Work out the finished part from the listing and answer in its coordinate system (mm). Face numbers are marked on the shaded views. Coordinates: 2 decimals unless noted, no trailing zeros. Order: outer loops, then holes, each group sorted by start corner. A loop starts at its lowest first (then second) coordinate and runs counter-clockwise, first axis right, second up. Notation, with made-up numbers: (15.5, 1) - (63.5, 1) arc R31 cw to (63.5, 34) - close; hole circle Ø1 at (-38.5, 39). An arc over 180 degrees is marked (long way). Answer as a JSON object with one key per item and string values. Group by question number.
1) Section B-B (z = 21) is taken. Give the vertices of the cut face in (x, y), plus the area to 3 significant figures.
2) The mould has two halves that part along X. Classify the marked faces 1, 2 and 3: released by +X, released by -X, zero draft, split by the parting line, or undercut.
3) Section A-A (y = -1.35) is taken. Give the vertices of the cut face in (x, z).
4) Each of these flat-tipped pins is pushed along its axis until it touches: P1, Ø4, axis at x = -9.5, z = -12, coming from the -Y side; P2, Ø1.2, axis at y = -2, z = 21.5, coming from the -X side; P3, Ø1, axis at x = -2.5, y = 0.5, coming from the -Z side. Where does it stop, or does it pass through?
5) Find the intervals of material crossed by line 1 along Y through (x, z) = (-11, -11); line 2 along X through (y, z) = (-2.3, 0); line 3 along Z through (x, y) = (-11, -1.35), in increasing order.
6) Section C-C (x = -17.75) is taken. Give the vertices of the cut face in (y, z), plus the area to 3 significant figures.
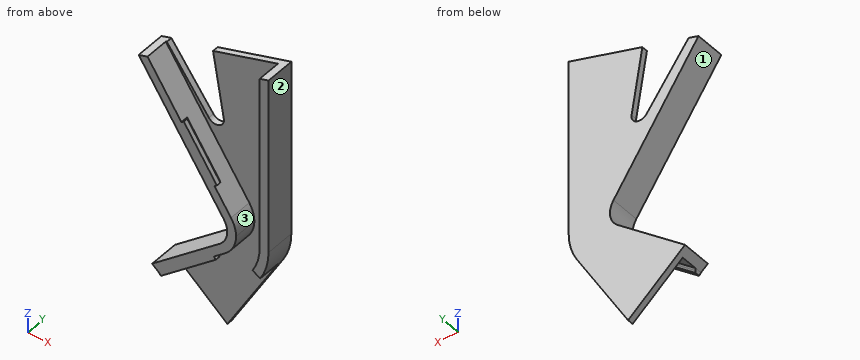
Autodesk Inventor part; units mm, degrees
ref_plane "YZ Plane" through (0, 0, 0) normal (1, 0, 0) x (0, 1, 0)
ref_plane "XZ Plane" through (0, 0, 0) normal (0, 1, 0) x (-1, 0, 0)
ref_plane "XY Plane" through (0, 0, 0) normal (0, 0, 1) x (1, 0, 0)
sketch "Sketch1" plane through (0, 0, 0) normal (0, 1, 0) x (-1, 0, 0)
  line L0 (0, 0) -> (0, 38)
  arc A0 (23.7631, 30.7092) -> (0, 38) centre (13, 38) ccw
  line L1 (0, 38) -> (13, 38)
  arc A1 (0, 0) -> (1.2058, -4.5) centre (9, 0) ccw
  line L2 (0, 0) -> (9, 0)
  line L3 (0, 0) -> (4, 0)
  arc A2 (4, 0) -> (5.8452, -3.8791) centre (9, 0) ccw
  arc A3 (4.8604, 2.8042) -> (4, 0) centre (9, 0) ccw
  line L4 (23.7631, 30.7092) -> (4.8604, 2.8042)
  line L5 (1.2058, -4.5) -> (12.7058, -24.4186)
  line L6 (12.7058, -24.4186) -> (17.9019, -21.4186)
  arc A4 (12.7058, -24.4186) -> (21.6877, -16.7637) centre (17.9019, -21.4186) ccw
  line L7 (5.8452, -3.8791) -> (21.6877, -16.7637)
  line L8 (20.5183, 23.2445) -> (6.1023, 1.9629)
  line L9 (18.2279, -12.0164) -> (6.7916, -2.7153)
  arc A5 (6.1023, 1.9629) -> (6.7916, -2.7153) centre (9, 0) ccw
  line L10 (-1.5, 30) -> (-1.5, 0)
  line L11 (8.567, -20.25) -> (-0.0933, -5.25)
  arc A6 (-1.5, 0) -> (-0.0933, -5.25) centre (9, 0) ccw
  line L12 (18.2279, -12.0164) -> (8.567, -20.25)
  line L13 (20.5183, 23.2445) -> (-1.5, 30)
  line L14 (4.8604, 2.8042) -> (19.0183, 23.7047)
  line L15 (0, 29.5398) -> (0, 0)
  line L16 (5.8452, -3.8791) -> (17.0671, -13.0058)
  line L17 (9.7278, -19.2607) -> (1.2058, -4.5)
  line L18 (1.2058, -4.5) -> (-0.0933, -5.25)
  dimension "d0" = 38
  dimension "d1" = 13
  dimension "d2" = 9
  dimension "d3" = 5
  dimension "d4" = 30
  dimension "d5" = 23
  dimension "d6" = 6
  dimension "d7" = 4
  dimension "d13" = 1.5
  dimension "d14" = 1.5
  dimension "d15" = 79.561
  dimension "d16" = 79.561
  dimension "d17" = 72.943
  dimension "d18" = 72.943
  dimension "d19" = 30
  dimension "d20" = 15
extrude "Extrusion1" add sketch "Sketch1" along normal blind 1 contours A1 L18 A6 L10 L13 L0 | L2 A2 L7 L12 L5 A1 | L0 L13 L4 A3 L2 | L5 L12 L11 L18 | A3 L4 L13 L8 A5 L2 | L2 A5 L9 L12 L7 A2
extrude "Extrusion2" add sketch "Sketch1" against normal blind 4 contours A1 L18 A6 L10 L13 L0 | A3 L4 L13 L8 A5 L2 | L2 A5 L9 L12 L7 A2
sketch "Sketch2" plane through (-5.8452, -4, -3.8791) normal (0.6309641, 0, -0.775812) x (-0.775812, 0, -0.6309641)
  line L0 (14.4647, 0) -> (0, 0)
  line L1 (14.4647, 0) -> (2.4647, 0)
  line L2 (2.4647, 1) -> (14.4647, 1)
  line L3 (14.4647, 4) -> (14.4647, 0)
  line L4 (14.4647, 0) -> (14.4647, 1)
  line L5 (2.4647, 1) -> (2.4647, 0)
  point P0 (-6.9823, 4)
  dimension "d28" = 12
extrude "Extrusion4" add sketch "Sketch2" along normal blind 0.5
sketch "Sketch3" plane through (-19.0183, -4, 23.7047) normal (0.8279279, 0, 0.5608345) x (0.5608345, 0, -0.8279279)
  line L0 (25.2444, 0) -> (0, 0)
  line L1 (20.2444, 0) -> (10.2444, 0)
  line L2 (10.2444, 1) -> (20.2444, 1)
  line L3 (20.2444, 1) -> (20.2444, 0)
  line L4 (10.2444, 1) -> (10.2444, 0)
  point P0 (30.2919, 4)
  dimension "d31" = 10
  dimension "d32" = 5
  dimension "d33" = 1
extrude "Extrusion5" add sketch "Sketch3" along normal blind 0.5
chamfer "Chamfer1" distance 0.25 angle 45 4 edges at (-12.4122, -3, -9.22) (-10.4687, -3, 11.0835) (-10.0547, -3, 11.3639) (-12.0967, -3, -9.6079)
sketch "Sketch4" plane through (0, 1, 0) normal (0, 1, 0) x (1, 0, 0)
  line L0 (-20.5183, -23.2445) -> (1.5, -30)
  line L1 (-18.8352, -23.7609) -> (-11.7144, -14.1579)
  arc A0 (-9.1763, -15.2361) -> (-11.7144, -14.1579) centre (-10.5752, -15.0026) ccw
  arc A1 (1.5, 0) -> (0.0933, 5.25) centre (-9, 0) ccw
  line L2 (0.0933, 5.25) -> (-10.567, 18.5455)
  line L3 (-8.567, 20.25) -> (-18.2279, 12.0164)
  line L4 (-10.567, 18.5455) -> (-8.567, 20.25)
  line L5 (-8.567, 20.25) -> (0.0933, 5.25)
  line L6 (-8.567, 20.25) -> (-10.567, 18.5455)
  line L7 (-9.1763, -15.2361) -> (-11, -26.1648)
  point P0 (0, 0)
  dimension "d42" = 2
extrude "Extrusion6" cut sketch "Sketch4" against normal blind 10 contours L1 A0 L7 L0
equation "\"d0\" = d8"
equation "\"d3\" = d2 - d7"
equation "\"d4\" = d9"
equation "\"d5\" = d10"
equation "\"d6\" = d11"
equation "\"d7\" = d12"
equation "\"d15\" = d16"
equation "\"d17\" = d18"
equation "\"d8\" = 38"
equation "\"d9\" = 30deg"
equation "\"d10\" = 23"
equation "\"d11\" = 6"
equation "\"d12\" = 4"
properties part number "flexible_leg_CS-3_V5_Armor"
Report:
{
 "1": {"outline": "(-19, -4) - (-17.19, -4) - (-17.19, 0) - (-16.79, 0) - (-16.79, 1) - (-19, 1) - close; (-10.14, 0) - (0, 0) - (0, -4) - (1.5, -4) - (1.5, 1) - (-10.14, 1) - close", "area": "27.1 mm²"},
 "2": {"face 1": "released by -X", "face 2": "released by +X", "face 3": "undercut"},
 "3": {"outline": "(-20.52, 23.24) - (-6.1, 1.96) arc R3.5 cw to (-6.79, -2.72) - (-18.23, -12.02) - (-17.07, -13.01) - (-5.85, -3.88) arc R5 ccw to (-4, 0) arc R5 ccw to (-4.86, 2.8) - (-19.02, 23.7) - close; (-1.21, -4.5) - (0.09, -5.25) arc R10.5 ccw to (1.5, 0) - (1.5, 30) - (0, 29.54) - (0, 0) arc R9 cw to start"},
 "4": {"P1": "stops at y = 0", "P2": "stops at x = -19.74", "P3": "stops at z = -10.61"},
 "5": {"line 1": "y = 0 to 1", "line 2": "x = -5.5 to -4, 0 to 1.5", "line 3": "z = -8.07 to -6.14, 9.19 to 11.87"},
 "6": {"outline": "(-4, -12.42) - (1, -12.42) - (1, -11.63) - (-4, -11.63) - close; (-4, 19.16) - (1, 19.16) - (1, 22.3) - (0, 22.3) - (0, 21.83) - (-4, 21.83) - close", "area": "17.8 mm²"}
}
